from build123d import *

# Parameters (mm, degrees)
EXTRUDE_2_DEPTH          = 15
CHAMFER_1_SIZE           = 5
CUT_EXTRUDE_START        = -13.418191
SKETCH_16_W              = 10.2
SKETCH_16_H              = 5.2
CUT_EXTRUDE_11_DEPTH     = 13.418191
SKETCH_17_W              = 10.2
SKETCH_17_H              = 5.2
CUT_EXTRUDE_12_DEPTH     = 15
SKETCH_19_R              = 2
CUT_EXTRUDE_13_DEPTH     = 83.70568747
CUT_EXTRUDE_14_REACH     = 104.544
SKETCH_21_R              = 2.5
SKETCH_24_R              = 2.032005788
CUT_EXTRUDE_16_DEPTH     = 10
PATTERN_LINEAR_1_COUNT   = 2
PATTERN_LINEAR_1_PITCH   = 20
CUT_EXTRUDE_20_REACH     = 84.706
SKETCH_31_R              = 2.5
MIRROR_1_COPY_1_SKETCH_R = 2.032005788
MIRROR_1_COPY_1_DEPTH    = 10
SKETCH_28_W              = 5.1
SKETCH_28_H              = 30.1
CUT_EXTRUDE_18_DEPTH     = 10
SKETCH_29_W              = 33.808551472
SKETCH_29_H              = 28.1
CUT_EXTRUDE_19_DEPTH     = 9


with BuildPart() as part:
    # Sketch 1 → Extrude 2 (new body)
    with BuildSketch(Plane.XY):
        Polygon((-15.918190797, 35), (-73.418190797, 35), (-73.418190797, 15), (-43.418190797, 15), (-43.418190797, -15), (-73.418190797, -15), (-73.418190797, -35), (-15.918190797, -35), align=None)
    extrude(amount=EXTRUDE_2_DEPTH)

    # Chamfer 1
    chamfer_1_edges = [part.edges().sort_by_distance(p)[0] for p in [
        (-73.418190797, 35, 7.5),
        (-15.918190797, 35, 7.5),
        (-15.918190797, -35, 7.5),
        (-73.418190797, -35, 7.5),
        (-43.418190797, -15, 7.5),
        (-43.418190797, 15, 7.5),
    ]]
    chamfer(chamfer_1_edges, length=CHAMFER_1_SIZE)

    # Sketch 16 → Cut-Extrude 11 (cut)
    with BuildSketch(Plane.ZY.offset(73.418190797).offset(CUT_EXTRUDE_START)):
        with Locations((7.5, 20)):
            Rectangle(SKETCH_16_W, SKETCH_16_H)
    cut_extrude_11 = extrude(amount=CUT_EXTRUDE_11_DEPTH, mode=Mode.SUBTRACT)

    # Sketch 17 → Cut-Extrude 12 (cut)
    with BuildSketch(Plane(origin=(-60, 0, 0), x_dir=(0, 0, -1), z_dir=(1, 0, 0))):
        with Locations((-7.5, 20)):
            Rectangle(SKETCH_17_W, SKETCH_17_H)
    cut_extrude_12 = extrude(amount=CUT_EXTRUDE_12_DEPTH, mode=Mode.SUBTRACT)

    # Sketch 19 → Cut-Extrude 13 (cut, through all)
    with BuildSketch(Plane.XY.offset(15)):
        with Locations((-45, 20)):
            Circle(SKETCH_19_R)
    cut_extrude_13 = extrude(amount=-CUT_EXTRUDE_13_DEPTH, mode=Mode.SUBTRACT)

    # Sketch 21 → Cut-Extrude 14 (cut, up to next)
    with BuildSketch(Plane(origin=(0, 35, 0), x_dir=(1, 0, 0), z_dir=(0, 1, 0)), mode=Mode.PRIVATE) as cut_extrude_14_sk1:
        with Locations(Location((-60, -7.5, 0), (0, 0, 270))):
            Circle(SKETCH_21_R)
    cut_extrude_14_tool1 = extrude(cut_extrude_14_sk1.sketch, amount=-CUT_EXTRUDE_14_REACH, mode=Mode.PRIVATE) & part.part
    cut_extrude_14 = cut_extrude_14_tool1.solids().sort_by_distance((-60, 35, 7.5))[0]
    add(cut_extrude_14, mode=Mode.SUBTRACT)

    # Sketch 24 → Cut-Extrude 16 (cut)
    with BuildSketch(Plane(origin=(0, 35, 0), x_dir=(1, 0, 0), z_dir=(0, 1, 0))):
        with Locations(Location((-50, -7.5, 0), (0, 0, 270))):
            Circle(SKETCH_24_R)
    cut_extrude_16 = extrude(amount=-CUT_EXTRUDE_16_DEPTH, mode=Mode.SUBTRACT)

    # Pattern Linear 1: Cut-Extrude 16 ×2
    with Locations(*[(i * PATTERN_LINEAR_1_PITCH, 0, 0) for i in range(1, PATTERN_LINEAR_1_COUNT)]):
        add(cut_extrude_16, mode=Mode.SUBTRACT)

    # Sketch 31 → Cut-Extrude 20 (cut, up to next)
    with BuildSketch(Plane.XY.offset(15), mode=Mode.PRIVATE) as cut_extrude_20_sk1:
        with Locations((-22.5, 29)):
            Circle(SKETCH_31_R)
    cut_extrude_20_tool1 = extrude(cut_extrude_20_sk1.sketch, amount=-CUT_EXTRUDE_20_REACH, mode=Mode.PRIVATE) & part.part
    # Sketch 31 → Cut-Extrude 20 (cut, up to next)
    with BuildSketch(Plane.XY.offset(15), mode=Mode.PRIVATE) as cut_extrude_20_sk2:
        with Locations((-67.5, 29)):
            Circle(SKETCH_31_R)
    cut_extrude_20_tool2 = extrude(cut_extrude_20_sk2.sketch, amount=-CUT_EXTRUDE_20_REACH, mode=Mode.PRIVATE) & part.part
    cut_extrude_20_1 = cut_extrude_20_tool1.solids().sort_by_distance((-22.5, 29, 15))[0]
    add(cut_extrude_20_1, mode=Mode.SUBTRACT)
    cut_extrude_20_2 = cut_extrude_20_tool2.solids().sort_by_distance((-67.5, 29, 15))[0]
    add(cut_extrude_20_2, mode=Mode.SUBTRACT)
    cut_extrude_20 = cut_extrude_20_1 + cut_extrude_20_2  # Cut-Extrude 20 as one shape, for the pattern or mirror that repeats it

    # Mirror 1: Cut-Extrude 11, Cut-Extrude 12, Cut-Extrude 13, Cut-Extrude 14, Cut-Extrude 16, Cut-Extrude 20 across plane
    add(cut_extrude_11.mirror(Plane.ZX), mode=Mode.SUBTRACT)
    add(cut_extrude_12.mirror(Plane.ZX), mode=Mode.SUBTRACT)
    add(cut_extrude_13.mirror(Plane.ZX), mode=Mode.SUBTRACT)
    add(cut_extrude_14.mirror(Plane.ZX), mode=Mode.SUBTRACT)
    add(cut_extrude_16.mirror(Plane.ZX), mode=Mode.SUBTRACT)
    add(cut_extrude_20.mirror(Plane.ZX), mode=Mode.SUBTRACT)

    # Mirror 1 copy 1 sketch → Mirror 1 copy 1 (cut)
    with BuildSketch(Plane(origin=(20, -35, 0), x_dir=(1, 0, 0), z_dir=(0, -1, 0))):
        with Locations((-50, 7.5)):
            Circle(MIRROR_1_COPY_1_SKETCH_R)
    extrude(amount=-MIRROR_1_COPY_1_DEPTH, mode=Mode.SUBTRACT)

    # Sketch 28 → Cut-Extrude 18 (cut)
    with BuildSketch(Plane.XY.offset(15)):
        with Locations((-21.502726402, 0)):
            Rectangle(SKETCH_28_W, SKETCH_28_H)
    extrude(amount=-CUT_EXTRUDE_18_DEPTH, mode=Mode.SUBTRACT)

    # Sketch 29 → Cut-Extrude 19 (cut)
    with BuildSketch(Plane.XY.offset(15)):
        with Locations((-40.957002138, 0)):
            Rectangle(SKETCH_29_W, SKETCH_29_H)
    extrude(amount=-CUT_EXTRUDE_19_DEPTH, mode=Mode.SUBTRACT)


solid = part.part
Geometry: final body of the model. Coordinates: model frame, mm. A direction names the side the tool comes from. Give positions to 0.01 mm unless a question says otherwise; leave off trailing zeros. Write each loop counter-clockwise with the first axis right and the second up, starting at its lowest first coordinate (ties: lowest second). Pieces come first, ordered by that corner, then holes. Notation, with made-up numbers: (28, 85) -> (79, 85) arc R16 ccw to (79, 115) -> close; hole circle Ø8 at (15, 65). An arc over 180 degrees is marked (long way). Answer as a JSON object with one key per item and string values.
1. Ray query, probe 1 along Y at (x, z) = (-22.5, 11.5); probe 2 along X at (y, z) = (-29, 11); probe 3 along Y at (x, z) = (-40.5, 8.75). Return the intervals inside material, ascending. Write a range as from..to.
Ans:
{"probe 1": "y = -35..-31.5, -26.5..-15.05, 15.05..26.5, 31.5..35", "probe 2": "x = -73.42..-70, -65..-25, -20..-15.92", "probe 3": "y = -35..-14.05, 14.05..35"}
2. Cut plane B-B on x = -61.5. Output: boundary loops of the cut face in (y, z), and give its area (3 significant figures).
Ans:
{"outline": "(-35, 0) -> (-15, 0) -> (-15, 15) -> (-35, 15) -> (-35, 9.5) -> (-22.6, 9.5) -> (-22.6, 12.6) -> (-17.4, 12.6) -> (-17.4, 2.4) -> (-22.6, 2.4) -> (-22.6, 5.5) -> (-35, 5.5) -> close; (15, 0) -> (35, 0) -> (35, 5.5) -> (22.6, 5.5) -> (22.6, 2.4) -> (17.4, 2.4) -> (17.4, 12.6) -> (22.6, 12.6) -> (22.6, 9.5) -> (35, 9.5) -> (35, 15) -> (15, 15) -> close", "area": "395 mm^2"}
3. Contact query for flat-ended pins moving along their axis: pin 1 (6.5 mm diameter, centred on x = -45, y = 20, fed in from +Z); pin 2 (0.7 mm diameter, centred on y = -18, z = 7.5, fed in from -X); pin 3 (3.5 mm diameter, centred on x = -50, z = 7.5, fed in from +Y); pin 4 (7 mm diameter, centred on x = -32.5, y = 1, fed in from +Z). Output: stop coordinate, or through.
Ans:
{"pin 1": "stops at z = 15", "pin 2": "stops at x = -45", "pin 3": "stops at y = 25", "pin 4": "stops at z = 6"}
4. Mould query, pull axis Y, two halves, no side actions, for faces 1 (the flat face through (-18.383, -32.465, 7.395)), 2 (the flat face through (-44, 35, 7)), 3 (the flat face through (-46.51, -13.09, 4.06)), 4 (the cylindrical face through (-51.984, 30.07, 7.06)). Classes: pulls with the +Y half, pulls with the -Y half, needs draft (parallel to the pull), parting line crosses it, or undercut.
Ans:
{"face 1": "pulls with the -Y half", "face 2": "pulls with the +Y half", "face 3": "undercut", "face 4": "needs draft"}
5. Cut plane C-C on z = 7.5. Count the separate pieces of the cut face and the enclosed holes in it, and give its area (3 significant figures).
Ans:
{"separate pieces": "3", "enclosed holes": "4", "area": "1,710 mm^2"}
6. Access query for faces 5 (the flat face through (-24.053, -0.1, 5.6)), 6 (the flat face through (-59, 22.6, 5)), 7 (the flat face through (-50, -25, 7)), 8 (the cylindrical face through (-31.8, 30.07, 8.44)). Directions: +Z, -Z, +X, -X, +Y, -Y. A direction counts if a zero-diameter tool reaches every point of the face in a straight line with its end or side. Return the directions, or none.
Ans:
{"face 5": "+Z", "face 6": "-X", "face 7": "-Y", "face 8": "+Y"}
7. Cut plane D-D on x = -67.5. Output: boundary loops of the cut face in (y, z), and give its area (3 significant figures).
Ans:
{"outline": "(-35, 0) -> (-31.5, 0) -> (-31.5, 15) -> (-35, 15) -> close; (-26.5, 0) -> (-15, 0) -> (-15, 15) -> (-26.5, 15) -> close; (15, 0) -> (26.5, 0) -> (26.5, 15) -> (15, 15) -> close; (31.5, 0) -> (35, 0) -> (35, 15) -> (31.5, 15) -> close; hole (-22.6, 2.4) -> (-17.4, 2.4) -> (-17.4, 12.6) -> (-22.6, 12.6) -> close; hole (17.4, 2.4) -> (22.6, 2.4) -> (22.6, 12.6) -> (17.4, 12.6) -> close", "area": "344 mm^2"}
8. Cut plane A-A on x = -55.5. Output: boundary loops of the cut face in (y, z).
Ans:
{"outline": "(-35, 0) -> (-15, 0) -> (-15, 15) -> (-35, 15) -> close; (15, 0) -> (35, 0) -> (35, 15) -> (15, 15) -> close; hole (-22.6, 2.4) -> (-17.4, 2.4) -> (-17.4, 12.6) -> (-22.6, 12.6) -> close; hole (17.4, 2.4) -> (22.6, 2.4) -> (22.6, 12.6) -> (17.4, 12.6) -> close"}
